```python
from build123d import *

# Parameters (mm, degrees)
SKETCH4_R      = 42.5
BASE_DEPTH     = 10
SKETCH5_R      = 5
SKETCH5_W      = 25
SKETCH5_H      = 40
TYRE_CUT_DEPTH = 10
SKETCH6_R      = 1.5
NUTS_DEPTH     = 10


with BuildPart() as part:
    # Sketch4 → base (new body)
    with BuildSketch(Plane.XY):
        Circle(SKETCH4_R)
    extrude(amount=BASE_DEPTH)

    # Sketch5 → Tyre cut (cut)
    with BuildSketch(Plane.XY):
        Circle(SKETCH5_R)
        with Locations((0, 40)):
            Rectangle(SKETCH5_W, SKETCH5_H)
        Polygon((11.070508076, -20.825317547), (23.570508076, 0.825317547), (58.211524227, -19.174682453), (45.711524227, -40.825317547), align=None)
        Polygon((-23.570508076, 0.825317547), (-11.070508076, -20.825317547), (-45.711524227, -40.825317547), (-58.211524227, -19.174682453), align=None)
    extrude(amount=TYRE_CUT_DEPTH, mode=Mode.SUBTRACT)

    # Sketch6 → NUTs (cut)
    with BuildSketch(Plane.XY):
        with Locations((7.71570735, 16)):
            Circle(SKETCH6_R)
        with Locations((7.71570735, 4.825317547)):
            Circle(SKETCH6_R)
        with Locations(Location((34.527154016, 4.825317547, 0), (0, 0, 180))):
            Circle(SKETCH6_R)
        with Locations(Location((34.527154016, 16, 0), (0, 0, 180))):
            Circle(SKETCH6_R)
        with Locations((9.998552785, -14.681998573)):
            Circle(SKETCH6_R)
        with Locations((0.320993902, -9.094657347)):
            Circle(SKETCH6_R)
        with Locations(Location((-13.084729431, -32.314051272, 0), (0, 0, 180))):
            Circle(SKETCH6_R)
        with Locations(Location((-3.407170547, -37.901392498, 0), (0, 0, 180))):
            Circle(SKETCH6_R)
        with Locations((-17.714260136, -1.318001427)):
            Circle(SKETCH6_R)
        with Locations((-8.036701252, 4.2693398)):
            Circle(SKETCH6_R)
        with Locations(Location((-21.442424585, 27.488733725, 0), (0, 0, 180))):
            Circle(SKETCH6_R)
        with Locations(Location((-31.119983469, 21.901392498, 0), (0, 0, 180))):
            Circle(SKETCH6_R)
    extrude(amount=NUTS_DEPTH, mode=Mode.SUBTRACT)


solid = part.part
```
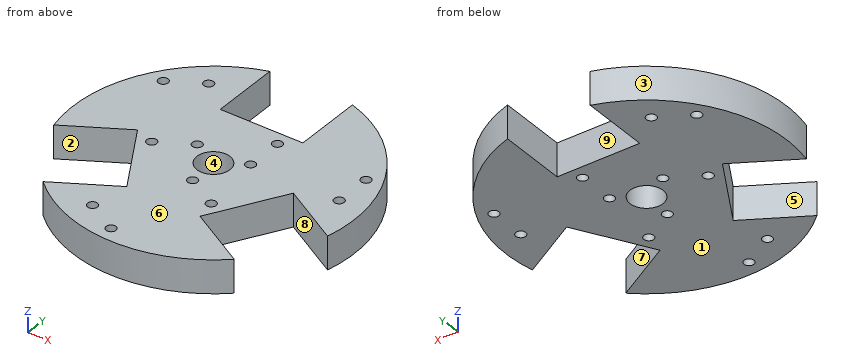
Geometry: final body of the model. Coordinates: model frame, mm. Face numbers are marked on the shaded views. A direction names the side the tool comes from. Coordinates: 2 decimals unless noted, no trailing zeros. Order: outer loops, then holes, each group sorted by start corner. A loop starts at its lowest first (then second) coordinate and runs counter-clockwise, first axis right, second up.
Item 1: Access query for the marked faces 5, 6, 7, 8 and 9. Directions: +Z, -Z, +X, -X, +Y, -Y. A direction counts if a zero-diameter tool reaches every point of the face in a straight line with its end or side. Return the directions, or none.
Answer:
face 5: +Z, -Z, -X
face 6: +Z, +X, -X, +Y, -Y
face 7: +Z, -Z, +X
face 8: +Z, -Z
face 9: +Z, -Z, +Y
Item 2: Material intervals for line 1 along Y through (x, z) = (9, 7); line 2 along Y through (x, z) = (-0.5, 2); line 3 along Y through (x, z) = (0, 3.5), sorted ascending.
Answer:
line 1: y = -41.54 to -15.8, -13.56 to 4.05, 5.6 to 15.23, 16.77 to 20
line 2: y = -42.5 to -10.35, -7.84 to -4.97, 4.97 to 20
line 3: y = -42.5 to -10.56, -7.63 to -5, 5 to 20
Item 3: Section query D-D (x = 19). Output: boundary loops of the cut face in (y, z).
Answer:
outline: (-38.02, 0) - (-25.4, 0) - (-25.4, 10) - (-38.02, 10) - close; (-7.09, 0) - (38.02, 0) - (38.02, 10) - (-7.09, 10) - close
Item 4: Section query B-B (x = -3). Output: boundary loops of the cut face in (y, z), then the cut area to 3 significant figures.
Answer:
outline: (-42.39, 0) - (-39.35, 0) - (-39.35, 10) - (-42.39, 10) - close; (-36.46, 0) - (-4, 0) - (-4, 10) - (-36.46, 10) - close; (4, 0) - (20, 0) - (20, 10) - (4, 10) - close
area: 515 mm2
Item 5: Section query A-A (y = 16). Output: boundary loops of the cut face in (x, z).
Answer:
outline: (-39.37, 0) - (6.22, 0) - (6.22, 10) - (-39.37, 10) - close; (9.22, 0) - (33.03, 0) - (33.03, 10) - (9.22, 10) - close; (36.03, 0) - (39.37, 0) - (39.37, 10) - (36.03, 10) - close
Item 6: Section query C-C (z = 5). State how many separate pieces and enclosed holes the cut face has, then the cut area to 3 significant figures.
Answer:
separate pieces: 1
enclosed holes: 13
area: 3,870 mm2
Item 7: Draft query along Y for the marked faces 1, 2, 3 and 4. Return one class per face: released by +Y, released by -Y, zero draft, split by the parting line, or undercut.
Answer:
face 1: zero draft
face 2: undercut
face 3: split by the parting line
face 4: undercut
Item 8: Contact query for flat-ended pins moving along their axis: P1, Ø2, axis at y = 31.5, z = 4.5, coming from the -X side; P2, Ø5, axis at x = 9, y = -4, coming from the -Z side; P3, Ø1, axis at y = -24, z = 2.5, coming from the +X side; P4, Ø3, axis at x = 6, z = 6.5, coming from the +Y side. Output: stop coordinate, or through.
Answer:
P1: stops at x = -29.6
P2: stops at z = 0
P3: stops at x = 17.44
P4: stops at y = 20
